Input: part model. Units: mm. Frame: model coordinates. Coordinates: 2 decimals unless noted, no trailing zeros. Write each loop counter-clockwise with the first axis right and the second up, starting at its lowest first coordinate (ties: lowest second). Pieces come first, ordered by that corner, then holes.
1) Section query A-A (x = 38.1). Output: boundary loops of the cut face in (y, z), then the cut area to 3 significant figures.
2) Section query B-B (y = -19.05). Output: boundary loops of the cut face in (x, z).
3) Line query: L1, parallel to X at y = 19, z = 3; L2, parallel to X at y = 39, z = 4.25; L3, parallel to X at y = -39.5, z = 5.75. Output: solid intervals per line, ascending.
4) Pin query (flat end, axial travel): pin 1 Ø11 at (x, y) = (52.39, 19.05) entering from -Z. Return the tip coordinate at first contact, or that it passes through.
5) Section query C-C (z = 4.5). State how many separate pieces and enclosed holes the cut face has, then the cut area to 3 significant figures.
from build123d import *

# Parameters (mm, degrees)
F0_W     = 304.8
F0_H     = 101.6
F1_DEPTH = 6.35
F2_R     = 4.78155
F3_DEPTH = 6.35
F4_R     = 4.78155
F5_DEPTH = 6.351


# Not quite as in the source:
# - a feature names something its author has since deleted; it is built from what else it names


with BuildPart() as f1:
    # F0 (on Top) → F1 (new body)
    with BuildSketch(Plane.XY):
        Rectangle(F0_W, F0_H)
    extrude(amount=F1_DEPTH)

    # F2 (on face) → F3 (cut, through all)
    with BuildSketch(Plane.XY.offset(6.35)):
        with Locations((-52.3875, 38.1)):
            Circle(F2_R)
        with Locations((52.3875, 38.1)):
            Circle(F2_R)
        with Locations((-52.3875, 19.05)):
            Circle(F2_R)
        with Locations((52.3875, 19.05)):
            Circle(F2_R)
        with Locations((-52.3875, 0)):
            Circle(F2_R)
        with Locations((-52.3875, -19.05)):
            Circle(F2_R)
        with Locations((-52.3875, -38.1)):
            Circle(F2_R)
        with Locations((52.3875, 0)):
            Circle(F2_R)
        with Locations((52.3875, -19.05)):
            Circle(F2_R)
        with Locations((52.3875, -38.1)):
            Circle(F2_R)
    extrude(amount=-F3_DEPTH, mode=Mode.SUBTRACT)

    # F4 (on face) → F5 (cut, through all)
    with BuildSketch(Plane.XY.offset(6.35)):
        with Locations((-38.1, 38.1)):
            Circle(F4_R)
        with Locations((38.1, 38.1)):
            Circle(F4_R)
    extrude(amount=-F5_DEPTH, mode=Mode.SUBTRACT)


solid = f1.part
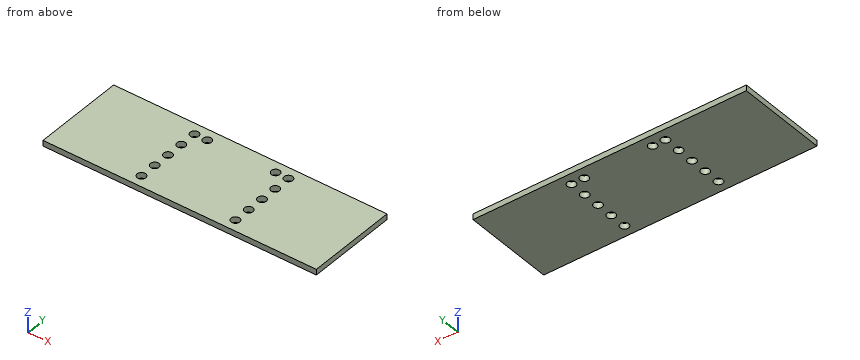
Answer:
1. outline: (-50.8, 0) - (33.32, 0) - (33.32, 6.35) - (-50.8, 6.35) - close; (42.88, 0) - (50.8, 0) - (50.8, 6.35) - (42.88, 6.35) - close
1. area: 584 mm2
2. outline: (-152.4, 0) - (-57.17, 0) - (-57.17, 6.35) - (-152.4, 6.35) - close; (-47.61, 0) - (47.61, 0) - (47.61, 6.35) - (-47.61, 6.35) - close; (57.17, 0) - (152.4, 0) - (152.4, 6.35) - (57.17, 6.35) - close
3. L1: x = -152.4 to -57.17, -47.61 to 47.61, 57.17 to 152.4
3. L2: x = -152.4 to -57.08, -47.69 to -42.8, -33.4 to 33.4, 42.8 to 47.69, 57.08 to 152.4
3. L3: x = -152.4 to -56.96, -47.82 to 47.82, 56.96 to 152.4
4. pin 1: stops at z = 0
5. separate pieces: 1
5. enclosed holes: 12
5. area: 30,100 mm2
